Autodesk Inventor part; units mm, degrees
ref_plane "YZ Plane" through (0, 0, 0) normal (1, 0, 0) x (0, 1, 0)
ref_plane "XZ Plane" through (0, 0, 0) normal (0, 1, 0) x (-1, 0, 0)
ref_plane "XY Plane" through (0, 0, 0) normal (0, 0, 1) x (1, 0, 0)
sketch "Sketch1" plane through (0, 0, 0) normal (0, 0, 1) x (1, 0, 0)
  line L0 (0, 0) -> (784.098, 0)
  line L1 (784.098, 0) -> (784.098, 655.574)
  line L2 (784.098, 655.574) -> (0, 655.574)
  line L3 (0, 655.574) -> (0, 0)
  dimension "d0" = 784.098
  dimension "d1" = 655.574
extrude "Extrusion1" add sketch "Sketch1" along normal blind 19.05
sketch "Sketch2" plane through (0, 0, 19.05) normal (0, 0, 1) x (1, 0, 0)
  line L0 (784.098, 0) -> (784.098, 655.574)
  line L1 (0, 0) -> (784.098, 0)
  line L2 (784.098, 0) -> (784.098, 655.574)
  line L3 (784.098, 655.574) -> (0, 655.574)
  line L4 (0, 655.574) -> (0, 0)
  line L5 (19.05, 636.524) -> (765.048, 636.524)
  line L6 (765.048, 636.524) -> (765.048, 19.05)
  line L7 (765.048, 19.05) -> (19.05, 19.05)
  line L8 (19.05, 19.05) -> (19.05, 636.524)
  dimension "d4" = 19.05
extrude "Extrusion2" add sketch "Sketch2" along normal blind 133.35
properties part number "Temporary Platform"
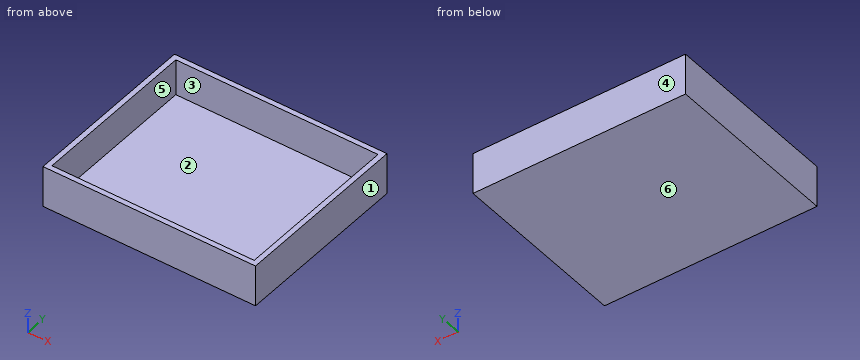
Design review of the part built by this model. Coordinates are the model's own, in mm. Face numbers are marked on the shaded views. A direction names the side the tool comes from. Coordinates: 2 decimals unless noted, no trailing zeros. Loops run counter-clockwise (first coordinate to the right, second up) from the corner with the lowest first, then second, coordinate; pieces in that order, holes last.
Item 1: Add section B-B (z = 125). Write out the cut boundary in (x, y), and give its area (3 significant figures).
Completed:
outline: (0, 0) - (784.1, 0) - (784.1, 655.57) - (0, 655.57) - close; hole (19.05, 19.05) - (765.05, 19.05) - (765.05, 636.52) - (19.05, 636.52) - close
area: 53,400 mm2
Item 2: Add section C-C (x = 86.5). Write out the cut boundary in (y, z), and give its area (3 significant figures).
Completed:
outline: (0, 0) - (655.57, 0) - (655.57, 152.4) - (636.52, 152.4) - (636.52, 19.05) - (19.05, 19.05) - (19.05, 152.4) - (0, 152.4) - close
area: 17,600 mm2
Item 3: Clearance check with a flat-ended pin moving along its axis: pin 1 (2 mm diameter, centred on y = 170, z = 80.5, fed in from -X). State where the tip first meets the part, or that it passes through.
Completed:
pin 1: stops at x = 0
Item 4: Add section A-A (y = 326.5). Write out the cut boundary in (x, z), and give its area (3 significant figures).
Completed:
outline: (0, 0) - (784.1, 0) - (784.1, 152.4) - (765.05, 152.4) - (765.05, 19.05) - (19.05, 19.05) - (19.05, 152.4) - (0, 152.4) - close
area: 20,000 mm2
Item 5: Wall thickness on L1, parallel to X at y = 530, z = 32.5; L2, parallel to Y at x = 567.5, z = 53; L3, parallel to Z at x = 661.5, y = 609: over which ranges is each line inside the solid? List them lowest first.
Completed:
L1: x = 0 to 19.05, 765.05 to 784.1
L2: y = 0 to 19.05, 636.52 to 655.57
L3: z = 0 to 19.05
Item 6: For the marked faces 5 and 6, list the 3-axis set-ups (+Z, -Z, +X, -X, +Y, -Y) from which the entire face can be reached by the end or side of a thin tool; tool diameter is ignored.
Completed:
face 5: +Z
face 6: -Z, +X, -X, +Y, -Y
Item 7: Draft analysis for pull direction Y (two halves, no side actions). For the marked faces 1, 2, 3 and 4, state which applies: pulls with the +Y half, pulls with the -Y half, needs draft (parallel to the pull), parting line crosses it, or undercut.
Completed:
face 1: needs draft
face 2: undercut
face 3: undercut
face 4: pulls with the +Y half
